Build history of the part. All positions in model axes, mm. Coordinates: 2 decimals unless noted, no trailing zeros. Write each question's results on one line, items separated by ' | '.
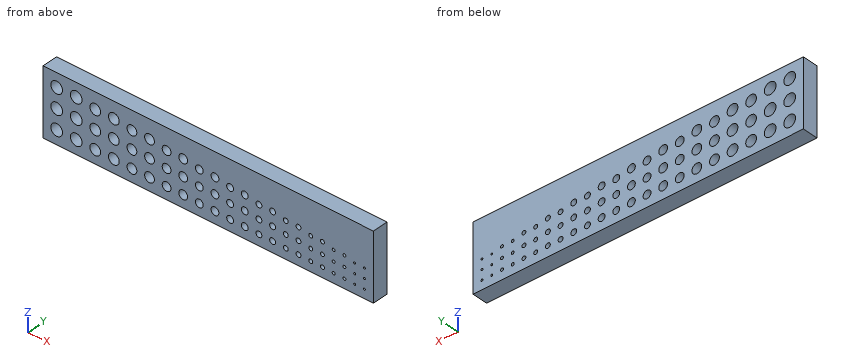
from build123d import *

# Parameters (mm, degrees)
F0_W     = 536.575
F0_H     = 107.95
F0_R     = 9.525
F0_R_2   = 8.7249
F0_R_3   = 7.1374
F0_R_4   = 7.9375
F0_R_5   = 6.35
F0_R_6   = 5.5499
F0_R_7   = 4.7625
F0_R_8   = 3.9624
F0_R_9   = 3.175
F0_R_10  = 2.3749
F0_R_11  = 1.5875
F1_DEPTH = 25.4


with BuildPart() as f1:
    # F0 (on Front) → F1 (new body)
    with BuildSketch(Plane.XZ):
        with Locations((38.201627, 15.935042)):
            Rectangle(F0_W, F0_H)
        with Locations((-207.860873, -15.814958)):
            Circle(F0_R, mode=Mode.SUBTRACT)
        with Locations((-176.110873, -15.814958)):
            Circle(F0_R, mode=Mode.SUBTRACT)
        with Locations((-145.171316, -16.615058)):
            Circle(F0_R_2, mode=Mode.SUBTRACT)
        with Locations((-115.021516, -16.615058)):
            Circle(F0_R_2, mode=Mode.SUBTRACT)
        with Locations((-29.331302, -18.202558)):
            Circle(F0_R_3, mode=Mode.SUBTRACT)
        with Locations((-85.669676, -17.402458)):
            Circle(F0_R_4, mode=Mode.SUBTRACT)
        with Locations((-57.094676, -17.402458)):
            Circle(F0_R_4, mode=Mode.SUBTRACT)
        with Locations((-2.356502, -18.202558)):
            Circle(F0_R_3, mode=Mode.SUBTRACT)
        with Locations((23.819057, -18.989958)):
            Circle(F0_R_5, mode=Mode.SUBTRACT)
        with Locations((-207.860873, 15.935042)):
            Circle(F0_R, mode=Mode.SUBTRACT)
        with Locations((-176.110873, 15.935042)):
            Circle(F0_R, mode=Mode.SUBTRACT)
        with Locations((-145.171316, 13.534742)):
            Circle(F0_R_2, mode=Mode.SUBTRACT)
        with Locations((-115.021516, 13.534742)):
            Circle(F0_R_2, mode=Mode.SUBTRACT)
        with Locations((-29.331302, 8.772242)):
            Circle(F0_R_3, mode=Mode.SUBTRACT)
        with Locations((-85.669676, 11.172542)):
            Circle(F0_R_4, mode=Mode.SUBTRACT)
        with Locations((-57.094676, 11.172542)):
            Circle(F0_R_4, mode=Mode.SUBTRACT)
        with Locations((-2.356502, 8.772242)):
            Circle(F0_R_3, mode=Mode.SUBTRACT)
        with Locations((23.819057, 6.410042)):
            Circle(F0_R_5, mode=Mode.SUBTRACT)
        with Locations((49.219057, -18.989958)):
            Circle(F0_R_5, mode=Mode.SUBTRACT)
        with Locations((73.805942, -19.790058)):
            Circle(F0_R_6, mode=Mode.SUBTRACT)
        with Locations((97.605742, -19.790058)):
            Circle(F0_R_6, mode=Mode.SUBTRACT)
        with Locations((120.604667, -20.577458)):
            Circle(F0_R_7, mode=Mode.SUBTRACT)
        with Locations((164.239623, -21.377558)):
            Circle(F0_R_8, mode=Mode.SUBTRACT)
        with Locations((142.829667, -20.577458)):
            Circle(F0_R_7, mode=Mode.SUBTRACT)
        with Locations((184.864423, -21.377558)):
            Circle(F0_R_8, mode=Mode.SUBTRACT)
        with Locations((204.686189, -22.164958)):
            Circle(F0_R_9, mode=Mode.SUBTRACT)
        with Locations((223.736189, -22.164958)):
            Circle(F0_R_9, mode=Mode.SUBTRACT)
        with Locations((241.968542, -22.965058)):
            Circle(F0_R_10, mode=Mode.SUBTRACT)
        with Locations((259.418342, -22.965058)):
            Circle(F0_R_10, mode=Mode.SUBTRACT)
        with Locations((276.062127, -23.752458)):
            Circle(F0_R_11, mode=Mode.SUBTRACT)
        with Locations((291.937127, -23.752458)):
            Circle(F0_R_11, mode=Mode.SUBTRACT)
        with Locations((120.604667, 1.647542)):
            Circle(F0_R_7, mode=Mode.SUBTRACT)
        with Locations((142.829667, 1.647542)):
            Circle(F0_R_7, mode=Mode.SUBTRACT)
        with Locations((164.239623, -0.752758)):
            Circle(F0_R_8, mode=Mode.SUBTRACT)
        with Locations((49.219057, 6.410042)):
            Circle(F0_R_5, mode=Mode.SUBTRACT)
        with Locations((73.805942, 4.009742)):
            Circle(F0_R_6, mode=Mode.SUBTRACT)
        with Locations((97.605742, 4.009742)):
            Circle(F0_R_6, mode=Mode.SUBTRACT)
        with Locations((204.686189, -3.114958)):
            Circle(F0_R_9, mode=Mode.SUBTRACT)
        with Locations((184.864423, -0.752758)):
            Circle(F0_R_8, mode=Mode.SUBTRACT)
        with Locations((223.736189, -3.114958)):
            Circle(F0_R_9, mode=Mode.SUBTRACT)
        with Locations((241.968542, -5.515258)):
            Circle(F0_R_10, mode=Mode.SUBTRACT)
        with Locations((259.418342, -5.515258)):
            Circle(F0_R_10, mode=Mode.SUBTRACT)
        with Locations((276.062127, -7.877458)):
            Circle(F0_R_11, mode=Mode.SUBTRACT)
        with Locations((291.937127, -7.877458)):
            Circle(F0_R_11, mode=Mode.SUBTRACT)
        with Locations((204.686189, 15.935042)):
            Circle(F0_R_9, mode=Mode.SUBTRACT)
        with Locations((223.736189, 15.935042)):
            Circle(F0_R_9, mode=Mode.SUBTRACT)
        with Locations((276.062127, 7.997542)):
            Circle(F0_R_11, mode=Mode.SUBTRACT)
        with Locations((291.937127, 7.997542)):
            Circle(F0_R_11, mode=Mode.SUBTRACT)
        with Locations((241.968542, 11.934542)):
            Circle(F0_R_10, mode=Mode.SUBTRACT)
        with Locations((259.418342, 11.934542)):
            Circle(F0_R_10, mode=Mode.SUBTRACT)
        with Locations((-29.331302, 35.747042)):
            Circle(F0_R_3, mode=Mode.SUBTRACT)
        with Locations((-85.669676, 39.747542)):
            Circle(F0_R_4, mode=Mode.SUBTRACT)
        with Locations((-57.094676, 39.747542)):
            Circle(F0_R_4, mode=Mode.SUBTRACT)
        with Locations((-2.356502, 35.747042)):
            Circle(F0_R_3, mode=Mode.SUBTRACT)
        with Locations((23.819057, 31.810042)):
            Circle(F0_R_5, mode=Mode.SUBTRACT)
        with Locations((-207.860873, 47.685042)):
            Circle(F0_R, mode=Mode.SUBTRACT)
        with Locations((-176.110873, 47.685042)):
            Circle(F0_R, mode=Mode.SUBTRACT)
        with Locations((-145.171316, 43.684542)):
            Circle(F0_R_2, mode=Mode.SUBTRACT)
        with Locations((-115.021516, 43.684542)):
            Circle(F0_R_2, mode=Mode.SUBTRACT)
        with Locations((73.805942, 27.809542)):
            Circle(F0_R_6, mode=Mode.SUBTRACT)
        with Locations((97.605742, 27.809542)):
            Circle(F0_R_6, mode=Mode.SUBTRACT)
        with Locations((164.239623, 19.872042)):
            Circle(F0_R_8, mode=Mode.SUBTRACT)
        with Locations((120.604667, 23.872542)):
            Circle(F0_R_7, mode=Mode.SUBTRACT)
        with Locations((142.829667, 23.872542)):
            Circle(F0_R_7, mode=Mode.SUBTRACT)
        with Locations((49.219057, 31.810042)):
            Circle(F0_R_5, mode=Mode.SUBTRACT)
        with Locations((184.864423, 19.872042)):
            Circle(F0_R_8, mode=Mode.SUBTRACT)
    extrude(amount=F1_DEPTH)


solid = f1.part
1. Band-saw the part on A-A on y = -8.75. Give the number of separate pieces and of enclosed holes in the cut face, then the cut area to 3 significant figures.
Solved:
separate pieces: 1 | enclosed holes: 66 | area: 50,200 mm2
2. Probe line 1 (Z direction, x = -58, y = -17.75); line 2 (Z direction, x = 49.5, y = -9.5). List the from-to ranges inside material, lowest first.
Solved:
line 1: z = -38.04 to -25.29, -9.52 to 3.29, 19.06 to 31.86, 47.63 to 69.91 | line 2: z = -38.04 to -25.33, -12.65 to 0.07, 12.75 to 25.47, 38.15 to 69.91
3. Drop a flat-ended pin along its axis: pin 1 Ø11.5 at (x, z) = (-2.36, 8.77) entering from -Y. Give the stop position or say it passes through.
Solved:
pin 1: passes through
